```python
from build123d import *

# Parameters (mm, degrees)
SKETCH1_W           = 44
SKETCH1_H           = 160
BOSS_EXTRUDE1_DEPTH = 6.35
SKETCH2_R           = 1.6
CUT_EXTRUDE1_DEPTH  = 84.212514083
SKETCH3_R           = 2.1
CUT_EXTRUDE2_DEPTH  = 84.212514083


with BuildPart() as part:
    # Sketch1 → Boss-Extrude1 (new body)
    with BuildSketch(Plane(origin=(0, 0, 0), x_dir=(1, 0, 0), z_dir=(0, 1, 0))):
        Rectangle(SKETCH1_W, SKETCH1_H)
    extrude(amount=BOSS_EXTRUDE1_DEPTH)

    # Sketch2 → Cut-Extrude1 (cut, through all)
    with BuildSketch(Plane(origin=(0, 6.35, 0), x_dir=(1, 0, 0), z_dir=(0, 1, 0))):
        with Locations(Location((-18.475, 18.475, 0), (0, 0, 270))):
            Circle(SKETCH2_R)
        with Locations(Location((-18.475, -18.475, 0), (0, 0, 270))):
            Circle(SKETCH2_R)
        with Locations(Location((18.475, -18.475, 0), (0, 0, 270))):
            Circle(SKETCH2_R)
        with Locations(Location((18.475, 18.475, 0), (0, 0, 270))):
            Circle(SKETCH2_R)
        with Locations(Location((-18.475, 76, 0), (0, 0, 270))):
            Circle(SKETCH2_R)
        with Locations(Location((-18.475, 39.05, 0), (0, 0, 270))):
            Circle(SKETCH2_R)
        with Locations(Location((18.475, 39.05, 0), (0, 0, 270))):
            Circle(SKETCH2_R)
        with Locations(Location((18.475, 76, 0), (0, 0, 270))):
            Circle(SKETCH2_R)
        with Locations(Location((-18.475, -39.05, 0), (0, 0, 270))):
            Circle(SKETCH2_R)
        with Locations(Location((-18.475, -76, 0), (0, 0, 270))):
            Circle(SKETCH2_R)
        with Locations(Location((18.475, -76, 0), (0, 0, 270))):
            Circle(SKETCH2_R)
        with Locations(Location((18.475, -39.05, 0), (0, 0, 270))):
            Circle(SKETCH2_R)
    extrude(amount=-CUT_EXTRUDE1_DEPTH, mode=Mode.SUBTRACT)

    # Sketch3 → Cut-Extrude2 (cut, through all)
    with BuildSketch(Plane(origin=(0, 6.35, 0), x_dir=(1, 0, 0), z_dir=(0, 1, 0))):
        with Locations(Location((-10, 30, 0), (0, 0, 270))):
            Circle(SKETCH3_R)
        with Locations(Location((10, 30, 0), (0, 0, 270))):
            Circle(SKETCH3_R)
        with Locations(Location((-10, -30, 0), (0, 0, 270))):
            Circle(SKETCH3_R)
        with Locations(Location((10, -30, 0), (0, 0, 270))):
            Circle(SKETCH3_R)
    extrude(amount=-CUT_EXTRUDE2_DEPTH, mode=Mode.SUBTRACT)


solid = part.part
```
The listing builds one solid part. Answer for the finished solid, in the listing's coordinates (mm). Coordinates: 2 decimals unless noted, no trailing zeros. Loops run counter-clockwise (first coordinate to the right, second up) from the corner with the lowest first, then second, coordinate; pieces in that order, holes last. Notation, with made-up numbers: (51.5, 27) -> (89.5, 27) arc R28 cw to (89.5, 57) -> close; hole circle Ø8 at (62.5, -14). An arc over 180 degrees is marked (long way). Return JSON: item names as keys, results as strings. Group by question number.
(1) A cutting plane is placed at B-B on y = 1.75. Count the separate pieces of the cut face and the enclosed holes in it, and give its area (3 significant figures).
(2) A cutting plane is placed at A-A on z = -39.05. Write down the section's boundary in (x, y) (3 decimals), and give its area (3 significant figures).
(3) Find the intervals of material crossed by probe 1 along X at (y, z) = (3.75, 39.05) (3 decimals); probe 2 along X at (y, z) = (5, 30); probe 3 along Z at (x, y) = (9, 4.25), in increasing order. Write a range as from..to.
(4) Determine the mould class of faces 1 (the cylindrical face through (10.09, 3.22, 27.9)), 2 (the flat face through (0, 6.35, -1)), 3 (the flat face through (0, 3, 80)) for opening direction Z: released by +Z, released by -Z, zero draft, split by the parting line, or undercut.
(5) Given pin 1 Ø5.5 at (x, z) = (-10, -30) entering from +Y; pin 2 Ø1.9 at (x, z) = (-18.475, -39.05) entering from -Y, each flat-ended and moving along its own axis, determine where each tip first touches the part or whether it passes through.
(6) A cutting plane is placed at C-C on z = 30. Write down the section's boundary in (x, y), and give its area (3 significant figures).
The answers:
{
 "1": {"separate pieces": "1", "enclosed holes": "16", "area": "6,890 mm^2"},
 "2": {"outline": "(-22, 0) -> (-20.075, 0) -> (-20.075, 6.35) -> (-22, 6.35) -> close; (-16.875, 0) -> (16.875, 0) -> (16.875, 6.35) -> (-16.875, 6.35) -> close; (20.075, 0) -> (22, 0) -> (22, 6.35) -> (20.075, 6.35) -> close", "area": "239 mm^2"},
 "3": {"probe 1": "x = -22..-20.075, -16.875..16.875, 20.075..22", "probe 2": "x = -22..-12.1, -7.9..7.9, 12.1..22", "probe 3": "z = -80..-31.85, -28.15..28.15, 31.85..80"},
 "4": {"face 1": "undercut", "face 2": "zero draft", "face 3": "released by +Z"},
 "5": {"pin 1": "stops at y = 6.35", "pin 2": "passes through"},
 "6": {"outline": "(-22, 0) -> (-12.1, 0) -> (-12.1, 6.35) -> (-22, 6.35) -> close; (-7.9, 0) -> (7.9, 0) -> (7.9, 6.35) -> (-7.9, 6.35) -> close; (12.1, 0) -> (22, 0) -> (22, 6.35) -> (12.1, 6.35) -> close", "area": "226 mm^2"}
}
